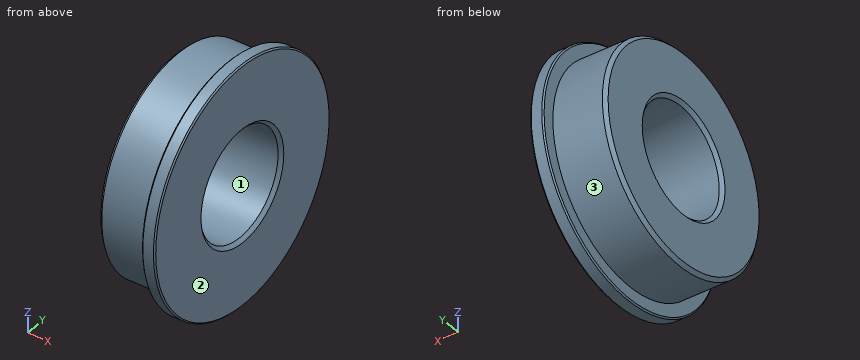
Autodesk Inventor part; units mm, degrees
ref_plane "YZ Plane" through (0, 0, 0) normal (1, 0, 0) x (0, 1, 0)
ref_plane "XZ Plane" through (0, 0, 0) normal (0, 1, 0) x (-1, 0, 0)
ref_plane "XY Plane" through (0, 0, 0) normal (0, 0, 1) x (1, 0, 0)
sketch "Skizze1" plane through (0, 0, 0) normal (0, 0, 1) x (1, 0, 0)
  line L0 (-18.8104, 0) -> (17.0467, 0)
  line L1 (-3.75, 4) -> (0.75, 4)
  line L2 (1, 4.25) -> (1, 8.9)
  line L3 (0.9, 9) -> (0.1, 9)
  line L4 (0, 8.9) -> (0, 8)
  line L5 (0, 8) -> (-3.75, 8)
  line L6 (-4, 7.75) -> (-4, 4.25)
  line L7 (-3.75, 8) -> (-4, 7.75)
  line L8 (-3.75, 4) -> (-4, 4.25)
  line L9 (0.75, 4) -> (1, 4.25)
  line L10 (0.1, 9) -> (0, 8.9)
  line L11 (1, 8.9) -> (0.9, 9)
  point P0 (0, 0)
  point P1 (-4, 4)
  point P2 (1, 4)
  point P3 (1, 9)
  point P4 (0, 9)
  point P5 (-4, 8)
  dimension "d0" = 5
  dimension "d1" = 18
  dimension "d2" = 1
  dimension "d3" = 16
  dimension "d4" = 8
  dimension "d5" = 0.25
  dimension "d6" = 0.25
  dimension "d7" = 0.25
  dimension "d8" = 0.25
  dimension "d9" = 0.25
  dimension "d10" = 0.25
  dimension "d11" = 0.1
  dimension "d12" = 0.1
  dimension "d13" = 0.1
  dimension "d14" = 0.1
revolve "Umdrehung1" add sketch "Skizze1" angle 360 about axis through (-18.8104, 0, 0) along (1, 0, 0)
properties part number "F688ZZ_V1" material "Stahl, Legierung"
Could you check a few things on this model? Use its own coordinates, in mm. Face numbers are marked on the shaded views. Give positions to 0.01 mm unless a question says otherwise; leave off trailing zeros. Order: outer loops, then holes, each group sorted by start corner. A loop starts at its lowest first (then second) coordinate and runs counter-clockwise, first axis right, second up. Notation, with made-up numbers: (-30, -17.75) -> (-13, -17.75) arc R16 ccw to (-13, -12.75) -> close; hole circle Ø6 at (2, 79.5). An arc over 180 degrees is marked (long way). Return JSON: item names as keys, results as strings.
1. Imagine slicing it at C-C on x = -0.75. List the corners of the cut face in (y, z) for me.
Answer list:
{"outline": "circle Ø16 at (0, 0); hole circle Ø8 at (0, 0)"}
2. Imagine slicing it at A-A on z = 0. List the corners of the cut face in (x, y) for me, then the cut area to 3 significant figures.
Answer list:
{"outline": "(-4, -7.75) -> (-3.75, -8) -> (0, -8) -> (0, -8.9) -> (0.1, -9) -> (0.9, -9) -> (1, -8.9) -> (1, -4.25) -> (0.75, -4) -> (-3.75, -4) -> (-4, -4.25) -> close; (-4, 4.25) -> (-3.75, 4) -> (0.75, 4) -> (1, 4.25) -> (1, 8.9) -> (0.9, 9) -> (0.1, 9) -> (0, 8.9) -> (0, 8) -> (-3.75, 8) -> (-4, 7.75) -> close", "area": "41.8 mm2"}
3. Thinking about a two-plate mould opening in Z: for the marked faces 1, 2 and 3, which applies, pulls with the +Z half, pulls with the -Z half, needs draft (parallel to the pull), parting line crosses it, or undercut?
Answer list:
{"face 1": "undercut", "face 2": "needs draft", "face 3": "parting line crosses it"}
4. For pin 1 Ø2 at (x, y) = (-2.5, 7) entering from -Z, with a flat end and sliding along its axis, tell me the tip position at first contact or that it passes through.
Answer list:
{"pin 1": "stops at z = -5.29"}
5. I need wall thicknesses on line 1 (Z direction, x = -0.2, y = 0); line 2 (Y direction, x = -1.5, z = 0.5); line 3 (Y direction, x = 0.65, z = -0.25). Which ranges of each line are inside material? Lowest first, please. Write a range as from..to.
Answer list:
{"line 1": "z = -8..-4, 4..8", "line 2": "y = -7.98..-3.97, 3.97..7.98", "line 3": "y = -9..-3.99, 3.99..9"}
